from build123d import *

# Parameters (mm, degrees)
F2_DEPTH = 5.08
F3_DEPTH = 12.7
F4_DEPTH = 12.7
F5_DEPTH = 12.7


# Not quite as in the source:
# - the program builds the solid bodies; features that only make, move or delete a surface that nothing else refers to are left out


with BuildPart() as f2:
    # F1 (on Front) → F2 (new body)
    with BuildSketch(Plane.XZ):
        Polygon((39.5757543065, 1.3013935037), (-0.0187108435, 21.5584816091), (2.2353688255, -22.8598751128), align=None)
    extrude(amount=F2_DEPTH)

    # F3 (add): a face of the model
    f3_faces = [f2.faces().sort_by_distance(p)[0] for p in [
        (1.108328991, -2.54, -0.6506967518),
    ]]
    extrude(f3_faces, amount=F3_DEPTH)

    # F4 (add): a face of the model
    f4_faces = [f2.faces().sort_by_distance(p)[0] for p in [
        (20.905561566, -2.54, -10.7792408046),
    ]]
    extrude(f4_faces, amount=F4_DEPTH)

    # F5 (add): a face of the model
    f5_faces = [f2.faces().sort_by_distance(p)[0] for p in [
        (19.7785217315, -2.54, 11.4299375564),
    ]]
    extrude(f5_faces, amount=F5_DEPTH)


solid = f2.part
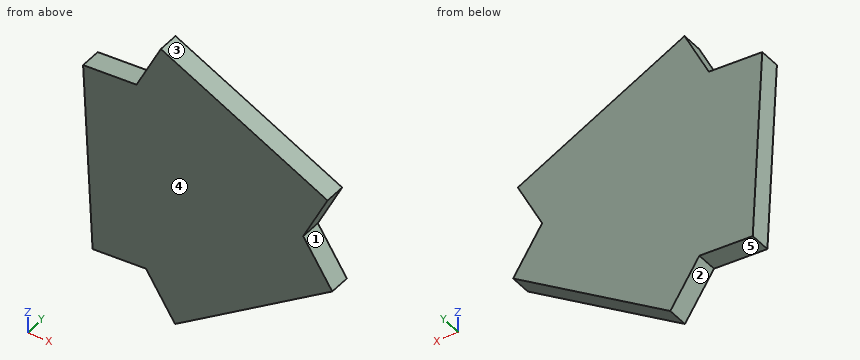
Geometry check sheet. Reference: the model listing, model coordinates, mm. Face numbers are marked on the shaded views. A direction names the side the tool comes from. Coordinates: 2 decimals unless noted, no trailing zeros. Order: outer loops, then holes, each group sorted by start corner. A loop starts at its lowest first (then second) coordinate and runs counter-clockwise, first axis right, second up. Notation, with made-up numbers: M 84.5,1.25 L 111.5,1.25 A22 ccw 111.5,8.25 Z; hole C 80,-23.75 d3. An arc over 180 degrees is marked long. Use CSV: the item, a comma, the result in double quotes.
Item 1: Cross-section at D-D on x = 29.5. Record the cut outline in (y, z), then the cut area to 3 significant figures.
Returned:
outline,"M -5.08,-20.34 L 0,-20.34 L 0,20.72 L -5.08,20.72 Z"
area,"209 mm2"
Item 2: Gauge pin test, flat ends, axial feed: pin 1 Ø1 at (x, y) = (7.5, -2.5) entering from +Z; pin 2 Ø1 at (x, y) = (28.5, -1) entering from +Z. Record the tip position at first contact, or that the pin passes through.
Returned:
pin 1,"stops at z = 32.23"
pin 2,"stops at z = 21.49"
Item 3: Thickness scan on line 1 along Z through (x, y) = (41, -1.7); line 2 along Z through (x, y) = (40.5, -2); line 3 along X through (y, z) = (-2.5, -0.5). Record the ranges inside material, lowest first.
Returned:
line 1,"z = -12.9 to -0.9, 4.09 to 14.84"
line 2,"z = -13.23 to -0.13, 3.11 to 15.09"
line 3,"x = -11.62 to 40.74"
Item 4: Cross-section at C-C on z = -1. Record the cut outline in (x, y).
Returned:
outline,"M -11.59,-5.08 L 41.06,-5.08 L 41.06,0 L -11.59,0 Z"
Item 5: Cross-section at A-A on x = 41. Record the cut outline in (y, z), then the cut area to 3 significant figures.
Returned:
outline,"M -5.08,-12.9 L 0,-12.9 L 0,-0.9 L -5.08,-0.9 Z; M -5.08,4.09 L 0,4.09 L 0,14.84 L -5.08,14.84 Z"
area,"116 mm2"
Item 6: Tool access check on the marked faces 4 and 5. Record the directions out of +Z, -Z, +X, -X, +Y, -Y that give a thin tool (end or side, any length) a straight path to the whole face; none if there is none.
Returned:
face 4,"+Z, -Z, +X, -X, -Y"
face 5,"-Z, +Y, -Y"
Item 7: Cross-section at B-B on y = -3.6. Record the cut outline in (x, z).
Returned:
outline,"M -12.7,20.91 L -10.45,-23.5 L 2.24,-22.86 L 9.13,-33.52 L 46.48,-9.36 L 39.58,1.3 L 45.36,12.61 L 5.77,32.86 L -0.02,21.56 Z"
Item 8: Mould release check, pull along Z, two halves, no side actions. Record for the marked faces 1, 2 and 3: pulls with the +Z half, pulls with the -Z half, needs draft (parallel to the pull), parting line crosses it, or undercut.
Returned:
face 1,"undercut"
face 2,"pulls with the -Z half"
face 3,"pulls with the +Z half"
